Geometry: final body of the model. Coordinates: model frame, mm. Coordinates: 2 decimals unless noted, no trailing zeros. Write each loop counter-clockwise with the first axis right and the second up, starting at its lowest first coordinate (ties: lowest second). Pieces come first, ordered by that corner, then holes. Notation, with made-up numbers: (-24, 51) -> (31, 51) arc R11 ccw to (31, 69) -> close; hole circle Ø7 at (-15.75, 18). An arc over 180 degrees is marked (long way). One line per item, written item: value.
Autodesk Inventor part; units mm, degrees
ref_plane "Work Plane2" through (-40, -40, 0) normal (0, 0, 1) x (1, 0, 0)
ref_plane "YZ Plane" through (0, 0, 0) normal (1, 0, 0) x (0, 1, 0)
ref_plane "XZ Plane" through (0, 0, 0) normal (0, 1, 0) x (-1, 0, 0)
ref_plane "Work Plane1" through (0, 0, 0) normal (0, 0, 1) x (1, 0, 0)
sketch "Sketch1" plane through (0, 0, 0) normal (0, 0, 1) x (1, 0, 0)
  circle A0 centre (0, 0) radius 40
  circle A1 centre (0, 0) radius 40
  circle A2 centre (37, 0) radius 1.4
  circle A3 centre (29.9336, 21.7481) radius 1.4
  circle A4 centre (11.4336, 35.1891) radius 1.4
  circle A5 centre (-11.4336, 35.1891) radius 1.4
  circle A6 centre (-29.9336, 21.7481) radius 1.4
  circle A7 centre (-37, 0) radius 1.4
  circle A8 centre (-29.9336, -21.7481) radius 1.4
  circle A9 centre (-11.4336, -35.1891) radius 1.4
  circle A10 centre (11.4336, -35.1891) radius 1.4
  circle A11 centre (29.9336, -21.7481) radius 1.4
  circle A12 centre (0, 0) radius 42
  circle A13 centre (0, 0) radius 18.5
  point P0 (0, 0)
  dimension "d9" = 2
extrude "Extrusion1" add sketch "Sketch1" along normal blind 3 contours A0 | A13
sketch "Sketch2" plane through (0, 0, 3) normal (0, 0, 1) x (1, 0, 0)
  circle A0 centre (0, 0) radius 40
  circle A1 centre (29.9336, -21.7481) radius 1.4
  circle A2 centre (11.4336, -35.1891) radius 1.4
  circle A3 centre (-11.4336, -35.1891) radius 1.4
  circle A4 centre (-29.9336, -21.7481) radius 1.4
  circle A5 centre (-37, 0) radius 1.4
  circle A6 centre (-29.9336, 21.7481) radius 1.4
  circle A7 centre (-11.4336, 35.1891) radius 1.4
  circle A8 centre (11.4336, 35.1891) radius 1.4
  circle A9 centre (29.9336, 21.7481) radius 1.4
  circle A10 centre (37, 0) radius 1.4
  point P0 (0, 0)
hole "Hole1" at (29.9336, 21.7481, 3) at (37, 0, 3) at (29.9336, -21.7481, 3) at (11.4336, -35.1891, 3) at (-11.4336, -35.1891, 3) at (-29.9336, -21.7481, 3) at (-37, 0, 3) at (-29.9336, 21.7481, 3) at (-11.4336, 35.1891, 3) at (11.4336, 35.1891, 3) direction (0, 0, -1) diameter 3.1 end through all
sketch "Sketch3" plane through (0, 0, 3) normal (0, 0, 1) x (1, 0, 0)
  circle A0 centre (0, 0) radius 40
  circle A1 centre (0, 0) radius 42
  point P0 (0, 0)
  dimension "d10" = 2
ref_plane "Work Plane2" through (-40, -40, 0) normal (0, 0, 1) x (1, 0, 0)
extrude "Extrusion2" add sketch "Sketch3" against normal up to surface (3 mm away)
sketch "Sketch4" plane through (0, 0, 3) normal (0, 0, 1) x (1, 0, 0)
  circle A0 centre (0, 0) radius 42
  circle A1 centre (-11.4336, 35.1891) radius 1.55
  circle A2 centre (-37, 0) radius 1.55
  circle A3 centre (-11.4336, -35.1891) radius 1.55
  circle A4 centre (29.9336, -21.7481) radius 1.55
  circle A5 centre (29.9336, 21.7481) radius 1.55
  circle A6 centre (37, 0) radius 1.55
  circle A7 centre (11.4336, -35.1891) radius 1.55
  circle A8 centre (-29.9336, -21.7481) radius 1.55
  circle A9 centre (-29.9336, 21.7481) radius 1.55
  circle A10 centre (11.4336, 35.1891) radius 1.55
  point P0 (0, 0)
properties part number "Anglerfish_Frontwindow_v0"
(1) Section D-D (x = 14.5). Return the cut outline in (y, z), then the cut area to 3 significant figures.
Responses:
outline: (-39.42, 0) -> (39.42, 0) -> (39.42, 3) -> (-39.42, 3) -> close
area: 237 mm2
(2) First-contact query: pin 1 (1 mm diameter, centred on y = -10, z = 2, fed in from -X). Flat tip, straight axial feed; report the tip coordinate or a pass-through.
Responses:
pin 1: stops at x = -40.91
(3) Section A-A (x = -37). Return the cut outline in (y, z).
Responses:
outline: (-19.87, 0) -> (-1.55, 0) -> (-1.55, 3) -> (-19.87, 3) -> close; (1.55, 0) -> (19.87, 0) -> (19.87, 3) -> (1.55, 3) -> close
(4) Section C-C (y = -31). Return the cut outline in (x, z), then the cut area to 3 significant figures.
Responses:
outline: (-28.34, 0) -> (28.34, 0) -> (28.34, 3) -> (-28.34, 3) -> close
area: 170 mm2
(5) Line query: line 1 (Y direction, x = -30.5, z = 1.55); line 2 (X direction, y = -22.5, z = 0.25); line 3 (Y direction, x = 29, z = 0.9). Output: solid intervals per line, ascending. Write a range as [from, to].
Responses:
line 1: y = [-28.87, -23.19], [-20.31, 20.31], [23.19, 28.87]
line 2: x = [-35.46, -31.29], [-28.58, 28.58], [31.29, 35.46]
line 3: y = [-30.38, -22.99], [-20.51, 20.51], [22.99, 30.38]
(6) Pull-direction query (X, two-part tool) for faces 1 (the cylindrical face through (40.06, 12.62, 1.52)), 2 (the cylindrical face through (-35.487, 0.336, 1.479)), 3 (the flat face through (-1, 1, 0)); classes: released by +X, released by -X, zero draft, split by the parting line, or undercut.
Responses:
face 1: split by the parting line
face 2: undercut
face 3: zero draft
(7) Section B-B (z = 1.05). State how many separate pieces and enclosed holes the cut face has, then the cut area to 3 significant figures.
Responses:
separate pieces: 1
enclosed holes: 10
area: 5,470 mm2
